```python
from build123d import *

# Parameters (mm, degrees)
F0_W     = 65
F0_H     = 30
F1_DEPTH = 1.5
F3_D     = 2.75
F4_R     = 3
F5_W     = 7.5
F5_H     = 4.7
F5_H_2   = 1
F6_DEPTH = 2.55
F5_W_2   = 11.25
F5_H_3   = 7
F5_H_4   = 0.5
F7_DEPTH = 3.3
F5_W_3   = 11.39
F5_H_5   = 12
F8_DEPTH = 1.47
F5_W_4   = 51.125
F5_H_6   = 5.375
F9_DEPTH = 2.5


with BuildPart() as f1:
    # F0 (on Top) → F1 (new body)
    with BuildSketch(Plane.XY):
        Rectangle(F0_W, F0_H)
    extrude(amount=F1_DEPTH)

    # F3 (through all)
    with Locations(Plane.XY.offset(1.5)):
        with Locations((-29, 11.5), (-29, -11.5), (29, -11.5), (29, 11.5)):
            Hole(F3_D / 2)

    # F4
    f4_edges = [f1.edges().sort_by_distance(p)[0] for p in [
        (-32.5, -15, 0.75),
        (-32.5, 15, 0.75),
        (32.5, -15, 0.75),
        (32.5, 15, 0.75),
    ]]
    fillet(f4_edges, radius=F4_R)

    # F5 (on face) → F6 (join)
    with BuildSketch(Plane.XY.offset(1.5)):
        with Locations((8.9, -12.65)):
            Rectangle(F5_W, F5_H)
        with Locations((8.9, -15.5)):
            Rectangle(F5_W, F5_H_2)
        with Locations((21.5, -15.5)):
            Rectangle(F5_W, F5_H_2)
        with Locations((21.5, -12.65)):
            Rectangle(F5_W, F5_H)
    extrude(amount=F6_DEPTH)

    # F5 (on face) → F7 (join)
    with BuildSketch(Plane.XY.offset(1.5)):
        with Locations((-20.1, -11.5)):
            Rectangle(F5_W_2, F5_H_3)
        with Locations((-20.1, -15.25)):
            Rectangle(F5_W_2, F5_H_4)
    extrude(amount=F7_DEPTH)

    # F5 (on face) → F8 (join)
    with BuildSketch(Plane.XY.offset(1.5)):
        with Locations((-25.155, 1.9)):
            Rectangle(F5_W_3, F5_H_5)
    extrude(amount=F8_DEPTH)

    # F5 (on face) → F9 (join)
    with BuildSketch(Plane.XY.offset(1.5)):
        with Locations((0, 11.5)):
            Rectangle(F5_W_4, F5_H_6)
    extrude(amount=F9_DEPTH)


solid = f1.part
```
Read the model definition and answer for the solid it produces. Units are mm, in the model's axes. A direction names the side the tool comes from. Give positions to 0.01 mm unless a question says otherwise; leave off trailing zeros. Order: outer loops, then holes, each group sorted by start corner. A loop starts at its lowest first (then second) coordinate and runs counter-clockwise, first axis right, second up. Notation, with made-up numbers: (-4.75, -7) -> (4.25, -7) arc R17 cw to (4.25, 3) -> close; hole circle Ø4 at (78.25, 35.25). An arc over 180 degrees is marked (long way). One line per item, written item: value. Start each with the question number.
(1) For a pull along X with two mould halves and no side action, classify faces 1 (the flat face through (25.562, 11, 3)), 2 (the cylindrical face through (30.374, 11.56, 0.74)), 3 (the flat face through (-25, -4.1, 2)) as released by +X, released by -X, zero draft, split by the parting line, or undercut.
(2) A tool of negligible diameter and unlimited length cuts with its end or side. For faces 4 (the flat face through (-19.46, 2, 2)), 5 (the flat face through (-25.562, 11, 3)), 6 (the flat face through (21, -13, 4.05)), 7 (the flat face through (17.75, -13, 3)), 8 (the flat face through (-25.725, -12, 3)), from which of +Z, -Z, +X, -X, +Y, -Y can it reach the whole face along a straight path? Write none if from no direction.
(3) Flat-ended cylindrical pins translate along their axes: P1, Ø0.8, axis at x = 9.5, y = -15.5, coming from the -Z side; P2, Ø1.6, axis at y = -0.5, z = 2.5, coming from the +X side; P3, Ø1.6, axis at x = -19, z = 2.5, coming from the +Y side. Find the tip coordinate at first contact, or state that the pin passes through.
(4) The part is cut by section C-C (y = 2.5). Determine the outline of the cut face in (x, z).
(5) The part is cut by section D-D (x = -5). Determine the outline of the cut face in (y, z), and give its area (3 significant figures).
(6) The part is cut by section B-B (x = 19.5). Determine the outline of the cut face in (y, z), and give its area (3 significant figures).
(7) The part is cut by section A-A (z = 0.8). Determine the outline of the cut face in (x, y) (3 decimals).
(8) Straight lines are drawn through the part: L1, parallel to Y at x = -29, z = 1 (3 decimals); L2, parallel to X at y = -15, z = 1.9 (3 decimals); L3, parallel to Y at x = -22, z = 1.7. For each, find the intervals that lie inside material, in ascending order.
Taken from the geometry:
1. face 1: released by +X
1. face 2: undercut
1. face 3: zero draft
2. face 4: +Z, +X
2. face 5: +Z, -X, +Y
2. face 6: +Z, +X, +Y, -Y
2. face 7: +Z, -Y
2. face 8: +Z, -X, -Y
3. P1: z = 1.5
3. P2: x = -19.46
3. P3: y = 14.19
4. outline: (-32.5, 0) -> (32.5, 0) -> (32.5, 1.5) -> (-19.46, 1.5) -> (-19.46, 2.97) -> (-30.85, 2.97) -> (-30.85, 1.5) -> (-32.5, 1.5) -> close
5. outline: (-15, 0) -> (15, 0) -> (15, 1.5) -> (14.19, 1.5) -> (14.19, 4) -> (8.81, 4) -> (8.81, 1.5) -> (-15, 1.5) -> close
5. area: 58.4 mm^2
6. outline: (-16, 1.5) -> (-15, 1.5) -> (-15, 0) -> (15, 0) -> (15, 1.5) -> (14.19, 1.5) -> (14.19, 4) -> (8.81, 4) -> (8.81, 1.5) -> (-10.3, 1.5) -> (-10.3, 4.05) -> (-16, 4.05) -> close
6. area: 73.0 mm^2
7. outline: (-32.5, -12) arc R3 ccw to (-29.5, -15) -> (29.5, -15) arc R3 ccw to (32.5, -12) -> (32.5, 12) arc R3 ccw to (29.5, 15) -> (-29.5, 15) arc R3 ccw to (-32.5, 12) -> close; hole circle Ø2.75 at (-29, -11.5); hole circle Ø2.75 at (-29, 11.5); hole circle Ø2.75 at (29, -11.5); hole circle Ø2.75 at (29, 11.5)
8. L1: -15 to -12.875, -10.125 to 10.125, 12.875 to 15
8. L2: -25.725 to -14.475, 5.15 to 12.65, 17.75 to 25.25
8. L3: -15.5 to -8, -4.1 to 7.9, 8.81 to 14.19
